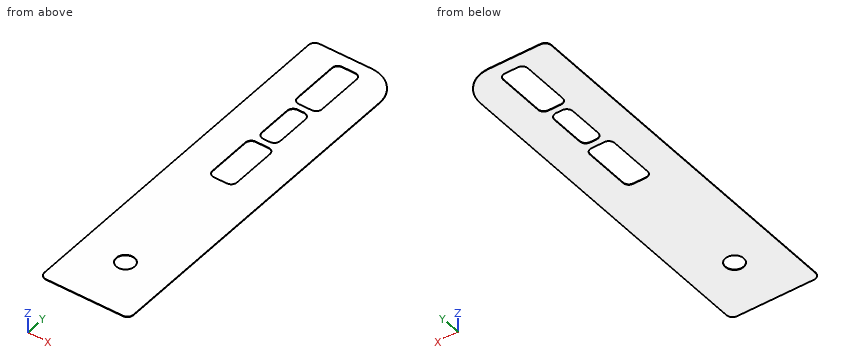
from build123d import *

# Parameters (mm, degrees)
BOSS_EXTRUDE5_DEPTH = 0.17
SKETCH1_R           = 3
CUT_EXTRUDE1_DEPTH  = 62.727456614
CUT_EXTRUDE2_DEPTH  = 62.727456614


with BuildPart() as part:
    # Sketch7 → Boss-Extrude5 (new body)
    with BuildSketch(Plane.XY):
        with BuildLine():
            Line((-12.5, 60), (4.5, 60))
            ThreePointArc((4.5, 60), (11.571067812, 57.071067812), (14.5, 50))
            Line((14.5, 50), (14.5, -58))
            ThreePointArc((14.5, -58), (13.914213562, -59.414213562), (12.5, -60))
            Line((12.5, -60), (-12.5, -60))
            ThreePointArc((-12.5, -60), (-13.914213562, -59.414213562), (-14.5, -58))
            Line((-14.5, -58), (-14.5, 58))
            ThreePointArc((-14.5, 58), (-13.914213562, 59.414213562), (-12.5, 60))
        make_face()
    extrude(amount=BOSS_EXTRUDE5_DEPTH)

    # Sketch1 (on Front Plane) → Cut-Extrude1 (cut, through all)
    with BuildSketch(Plane.XY):
        with Locations((0, -42)):
            Circle(SKETCH1_R)
        with BuildLine():
            Line((-2.1, -0.3), (2.1, -0.3))
            ThreePointArc((2.1, -0.3), (3.443502884, 0.256497116), (4, 1.6))
            Line((4, 1.6), (4, 16.031829774))
            ThreePointArc((4, 16.031829774), (3.443502884, 17.375332658), (2.1, 17.931829774))
            Line((2.1, 17.931829774), (-2.1, 17.931829774))
            ThreePointArc((-2.1, 17.931829774), (-3.443502884, 17.375332658), (-4, 16.031829774))
            Line((-4, 16.031829774), (-4, 1.6))
            ThreePointArc((-4, 1.6), (-3.443502884, 0.256497116), (-2.1, -0.3))
        make_face()
        with BuildLine():
            Line((2.1, 56), (-2.1, 56))
            ThreePointArc((-2.1, 56), (-3.443502884, 55.443502884), (-4, 54.1))
            Line((-4, 54.1), (-4, 38.9))
            ThreePointArc((-4, 38.9), (-3.443502884, 37.556497116), (-2.1, 37))
            Line((-2.1, 37), (2.1, 37))
            ThreePointArc((2.1, 37), (3.443502884, 37.556497116), (4, 38.9))
            Line((4, 38.9), (4, 54.1))
            ThreePointArc((4, 54.1), (3.443502884, 55.443502884), (2.1, 56))
        make_face()
    extrude(amount=CUT_EXTRUDE1_DEPTH, mode=Mode.SUBTRACT)

    # Sketch8 → Cut-Extrude2 (cut, through all)
    with BuildSketch(Plane.XY.offset(0.17)):
        with BuildLine():
            Line((-3, 33), (-3, 22))
            ThreePointArc((-3, 22), (-2.414213562, 20.585786438), (-1, 20))
            Line((-1, 20), (1, 20))
            ThreePointArc((1, 20), (2.414213562, 20.585786438), (3, 22))
            Line((3, 22), (3, 33))
            ThreePointArc((3, 33), (2.414213562, 34.414213562), (1, 35))
            Line((1, 35), (-1, 35))
            ThreePointArc((-1, 35), (-2.414213562, 34.414213562), (-3, 33))
        make_face()
    extrude(amount=-CUT_EXTRUDE2_DEPTH, mode=Mode.SUBTRACT)


solid = part.part
Part model, mm, in its own coordinate system. Give positions to 0.01 mm unless a question says otherwise; leave off trailing zeros. Loops run counter-clockwise (first coordinate to the right, second up) from the corner with the lowest first, then second, coordinate; pieces in that order, holes last. Notation, with made-up numbers: (84.25, 77.5) -> (125.25, 77.5) arc R34 ccw to (125.25, 108.5) -> close; hole circle Ø2 at (49, -34). An arc over 180 degrees is marked (long way). Write each question's results on one line, items separated by ' | '. Start each with the question number.
Q1. Band-saw the part on B-B on x = 0. List the corners of the cut face in (y, z).
Q2. Band-saw the part on A-A on y = -42. List the corners of the cut face in (x, z), plus the area to 3 significant figures.
Q3. Pin check, flat tip, straight feed: P1, Ø5, axis at x = 0, y = -42, coming from the +Z side. Stop position of the tip, or through.
Q4. Band-saw the part on C-C on z = 0.1. Count the separate pieces of the cut face and the enclosed holes in it, plus the area to 3 significant figures.
Q5. Wall check: L1, parallel to Y at x = 0, z = 0.1; L2, parallel to X at y = -42, z = 0.1; L3, parallel to Y at x = 2.5, z = 0.05. Give the ranges that are in metal, low to high.
Results are:
1) outline: (-60, 0) -> (-45, 0) -> (-45, 0.17) -> (-60, 0.17) -> close; (-39, 0) -> (-0.3, 0) -> (-0.3, 0.17) -> (-39, 0.17) -> close; (17.93, 0) -> (20, 0) -> (20, 0.17) -> (17.93, 0.17) -> close; (35, 0) -> (37, 0) -> (37, 0.17) -> (35, 0.17) -> close; (56, 0) -> (60, 0) -> (60, 0.17) -> (56, 0.17) -> close
2) outline: (-14.5, 0) -> (-3, 0) -> (-3, 0.17) -> (-14.5, 0.17) -> close; (3, 0) -> (14.5, 0) -> (14.5, 0.17) -> (3, 0.17) -> close | area: 3.91 mm²
3) P1: passes through
4) separate pieces: 1 | enclosed holes: 4 | area: 3,050 mm²
5) L1: y = -60 to -45, -39 to -0.3, 17.93 to 20, 35 to 37, 56 to 60 | L2: x = -14.5 to -3, 3 to 14.5 | L3: y = -60 to -43.66, -40.34 to -0.26, 17.89 to 20.68, 34.32 to 37.04, 55.96 to 60
